Answer from the drawing. Dimensions are ordinates in mm from the lowest x, y and z of the part. Coordinates: 2 decimals unless noted, no trailing zeros. Order: outer loops, then holes, each group sorted by start corner. A loop starts at its lowest first (then second) coordinate and runs counter-clockwise, first axis right, second up.
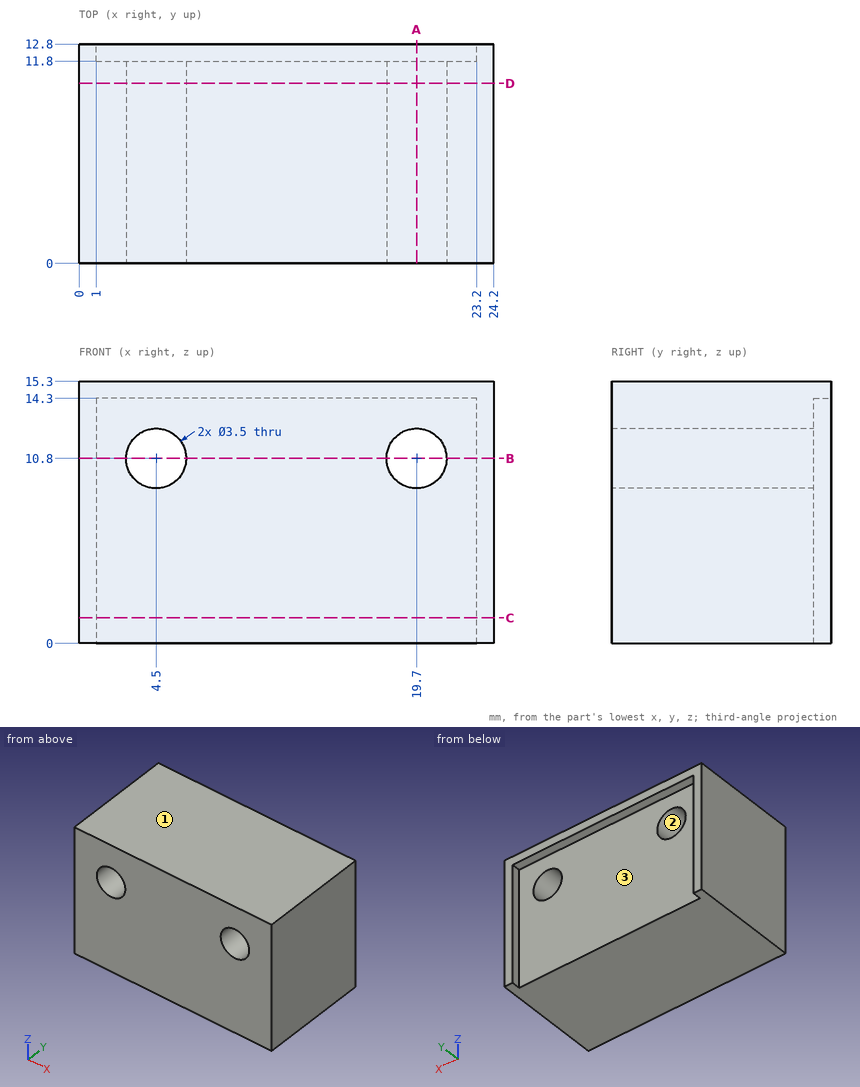
1) Section A-A (x = 19.7) is taken. Give the vertices of the cut face in (y, z), then the cut area to 3 significant figures.
2) Consider L1, parallel to X at y = 3.25, z = 10.8; L2, parallel to X at y = 12.25, z = 3.5; L3, parallel to Y at x = 17, z = 1.75. Determine where each line is inside the solid, lowest interval first.
3) Determine the mould class of the marked faces 1, 2 and 3 for opening direction Z: released by +Z, released by -Z, zero draft, split by the parting line, or undercut.
4) Section C-C (z = 1.5) is taken. Give the vertices of the cut face in (x, y), then the cut area to 3 significant figures.
5) Section D-D (y = 10.5) is taken. Give the vertices of the cut face in (x, z), then the cut area to 3 significant figures.
6) This flat-tipped pin is pushed along its axis until it touches: P1, Ø4, axis at x = 19.7, z = 10.8, coming from the +Y side. Where does it stop, or does it pass through?
7) Section B-B (z = 10.8) is taken. Give the vertices of the cut face in (x, y).
Filled sheet:
1. outline: (0, 0) - (11.8, 0) - (11.8, 9.05) - (0, 9.05) - close; (0, 12.55) - (11.8, 12.55) - (11.8, 14.3) - (12.8, 14.3) - (12.8, 15.3) - (0, 15.3) - close
1. area: 140 mm2
2. L1: x = 0 to 2.75, 6.25 to 17.95, 21.45 to 24.2
2. L2: x = 0 to 1, 23.2 to 24.2
2. L3: y = 0 to 11.8
3. face 1: released by +Z
3. face 2: undercut
3. face 3: zero draft
4. outline: (0, 0) - (24.2, 0) - (24.2, 12.8) - (23.2, 12.8) - (23.2, 11.8) - (1, 11.8) - (1, 12.8) - (0, 12.8) - close
4. area: 288 mm2
5. outline: (0, 0) - (24.2, 0) - (24.2, 15.3) - (0, 15.3) - close; hole circle Ø3.5 at (4.5, 10.8); hole circle Ø3.5 at (19.7, 10.8)
5. area: 351 mm2
6. P1: stops at y = 11.8
7. outline: (0, 0) - (2.75, 0) - (2.75, 11.8) - (1, 11.8) - (1, 12.8) - (0, 12.8) - close; (6.25, 0) - (17.95, 0) - (17.95, 11.8) - (6.25, 11.8) - close; (21.45, 0) - (24.2, 0) - (24.2, 12.8) - (23.2, 12.8) - (23.2, 11.8) - (21.45, 11.8) - close
